The drawing under review shows one solid part. Ordinate dimensions are in mm from its lowest x, y, z. Coordinates: 2 decimals unless noted, no trailing zeros. Write each loop counter-clockwise with the first axis right and the second up, starting at its lowest first coordinate (ties: lowest second). Pieces come first, ordered by that corner, then holes.
Q1. Insertion check: pin 1 (1.8 mm diameter, centred on x = 8, z = 16.25, fed in from +Y). The pin has a flat end and moves straight along its axis. Give the tip position at first contact, or say it passes through.
Q2. Take a section at C-C (y = 0.55). Give the boundary of the cut face in (x, z), and give its area (3 significant figures).
Q3. For probe 1 along Z at (x, y) = (21.8, 1.1); probe 2 along X at (y, z) = (0.9, 16.25), list the stretches that pass through material, from the lowest coordinate up.
Q4. Take a section at B-B (z = 16.25). Give the boundary of the cut face in (x, y).
Q5. Take a section at A-A (x = 8). Give the boundary of the cut face in (y, z), and give its area (3 significant figures).
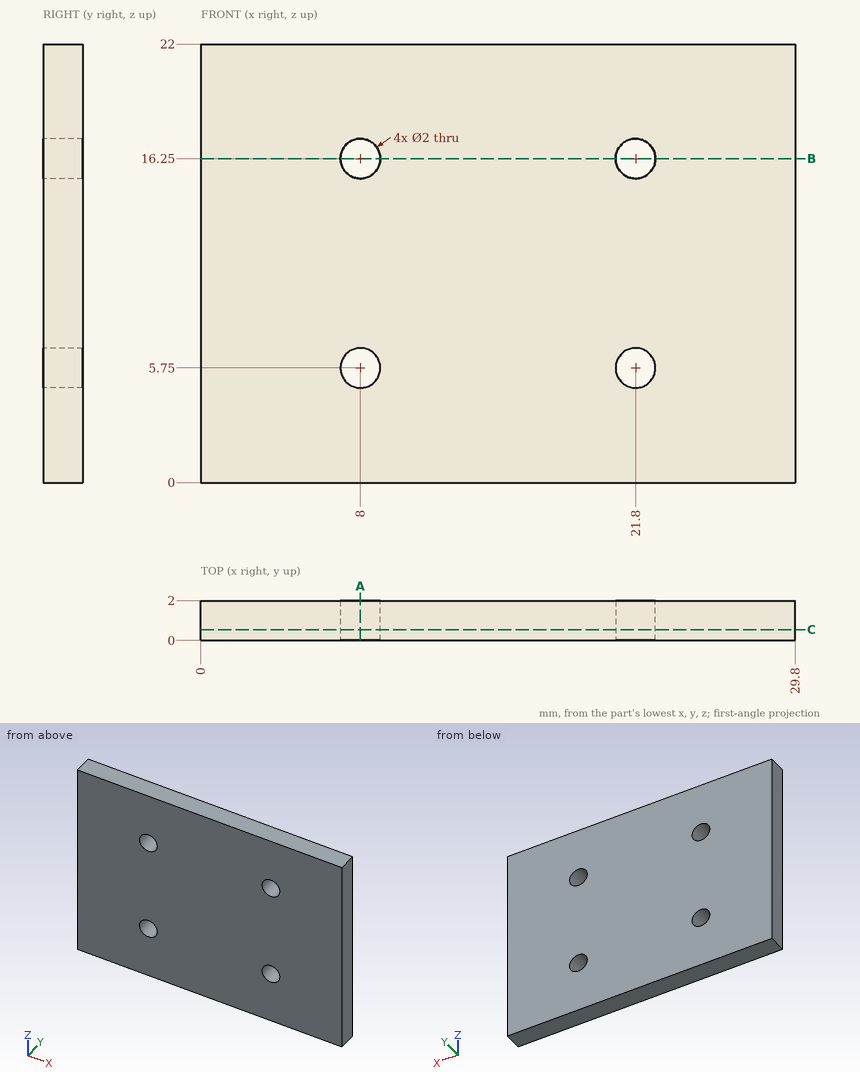
Response:
1. pin 1: passes through
2. outline: (0, 0) - (29.8, 0) - (29.8, 22) - (0, 22) - close; hole circle Ø2 at (8, 5.75); hole circle Ø2 at (8, 16.25); hole circle Ø2 at (21.8, 5.75); hole circle Ø2 at (21.8, 16.25)
2. area: 643 mm2
3. probe 1: z = 0 to 4.75, 6.75 to 15.25, 17.25 to 22
3. probe 2: x = 0 to 7, 9 to 20.8, 22.8 to 29.8
4. outline: (0, 0) - (7, 0) - (7, 2) - (0, 2) - close; (9, 0) - (20.8, 0) - (20.8, 2) - (9, 2) - close; (22.8, 0) - (29.8, 0) - (29.8, 2) - (22.8, 2) - close
5. outline: (0, 0) - (2, 0) - (2, 4.75) - (0, 4.75) - close; (0, 6.75) - (2, 6.75) - (2, 15.25) - (0, 15.25) - close; (0, 17.25) - (2, 17.25) - (2, 22) - (0, 22) - close
5. area: 36.0 mm2
